For this review, take the finished solid that the model builds, in its own axes (mm). Face numbers are marked on the shaded views. A direction names the side the tool comes from. Coordinates: 2 decimals unless noted, no trailing zeros. Loops run counter-clockwise (first coordinate to the right, second up) from the corner with the lowest first, then second, coordinate; pieces in that order, holes last. Notation, with made-up numbers: (-12.5, 8.5) - (37.5, 8.5) arc R20 cw to (37.5, 40.5) - close; hole circle Ø6 at (8.5, 7.5). An arc over 180 degrees is marked (long way). Use one line per item in the form item = value. Start each with the question number.
1. Machinability: for the marked faces 1 and 2, which of the approach directions +Z, -Z, +X, -X, +Y, -Y give a long, thin tool a straight path to every point of the face, cutting with its end or side? Answer none if there is none.
2. Add section C-C on x = 31.5. Give the boundary of the cut face in (y, z) (1 decimal), and give its area (3 significant figures).
3. To check wall thickness, follow probe 1 along X at (y, z) = (3, 17.5); probe 2 along Y at (x, z) = (-0.5, 3.5) (1 decimal); probe 3 along Z at (x, y) = (24.5, -21.5) (3 decimals). State the ranges of each line that lie inside material, in increasing order.
4. Draft analysis for pull direction X (two halves, no side actions). For the marked faces 3, 4 and 5, state which applies: +X half, -X half, draft (parallel to the pull), parting line (faces both ways), or undercut.
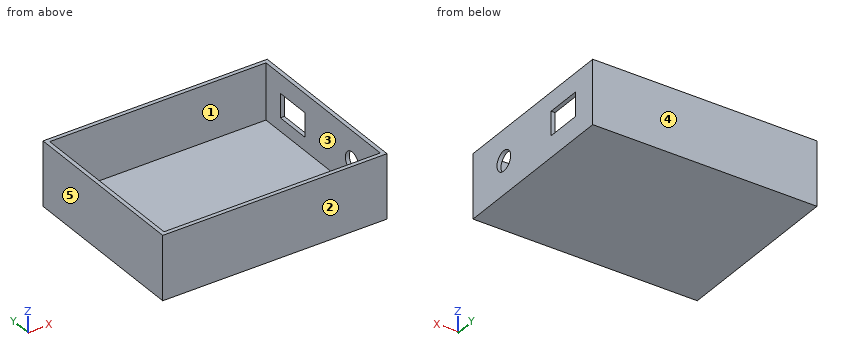
```python
from build123d import *

# Parameters (mm, degrees)
F0_W     = 88.9
F0_H     = 69.85
F0_W_2   = 85.725
F0_H_2   = 66.675
F1_DEPTH = 25.4
F2_DEPTH = 3.175
F4_D     = 7.9502
F4_DEPTH = 12.7
F3_W     = 14.2875
F3_H     = 9.525
F5_DEPTH = 1.5875


with BuildPart() as f1:
    # F0 (on Top) → F1 (new body)
    with BuildSketch(Plane.XY):
        Rectangle(F0_W, F0_H)
        Rectangle(F0_W_2, F0_H_2, mode=Mode.SUBTRACT)
    extrude(amount=F1_DEPTH)

    # F0 (on Top) → F2 (join)
    with BuildSketch(Plane.XY):
        Rectangle(F0_W_2, F0_H_2)
    extrude(amount=F2_DEPTH)

    # F4
    with Locations(Plane.YZ.offset(44.45)):
        with Locations((-16.949601, 13.195173)):
            Hole(F4_D / 2, depth=F4_DEPTH)

    # F3 (on face) → F5 (cut, through all)
    with BuildSketch(Plane.YZ.offset(44.45)):
        with Locations((17.784979, 13.195173)):
            Rectangle(F3_W, F3_H)
    extrude(amount=-F5_DEPTH, mode=Mode.SUBTRACT)


solid = f1.part
```
Conclusion:
q1.face_1 = +Z
q1.face_2 = +Z, -Z, +X, -X, -Y
q2.outline = (-34.9, 0) - (34.9, 0) - (34.9, 25.4) - (33.3, 25.4) - (33.3, 3.2) - (-33.3, 3.2) - (-33.3, 25.4) - (-34.9, 25.4) - close
q2.area = 292 mm^2
q3.probe_1 = -44.45 to -42.86, 42.86 to 44.45
q3.probe_2 = -34.9 to -33.3, 33.3 to 34.9
q3.probe_3 = 0 to 3.175
q4.face_3 = undercut
q4.face_4 = draft
q4.face_5 = -X half
